For this review, use the dimensioned drawing (mm, ordinates from the lowest corner) and the shaded views. A direction names the side the tool comes from. Give positions to 0.01 mm unless a question says otherwise; leave off trailing zeros. Write each loop counter-clockwise with the first axis right and the second up, starting at its lowest first coordinate (ties: lowest second). Pieces come first, ordered by that corner, then holes. Notation, with made-up numbers: M 61.5,-3.5 L 90.5,-3.5 A15 ccw 90.5,6.5 Z; hole C 36.5,50 d9. An arc over 180 degrees is marked long. One line per item, written item: value. Start each with the question number.
Item 1: Consider section A-A, the plane x = 24. Write out the cut boundary in (y, z).
Item 2: Consider section D-D, the plane y = 47. Write out the cut boundary in (x, z).
Item 3: Clearance check with flat-ended pins moving along their axes: pin 1 Ø1.5 at (x, z) = (61, 39.5) entering from +Y; pin 2 Ø1 at (y, z) = (48.5, 64) entering from +X; pin 3 Ø8 at (x, y) = (54, 46) entering from +Z; pin 4 Ø8 at (x, z) = (66, 65) entering from -Y. State where each tip first meets the part, or that it passes through.
Item 4: Consider section B-B, the plane z = 16.5. Write out the cut boundary in (x, y).
Item 5: To check wall thickness, follow probe 1 along Z at (x, y) = (66, 22); probe 2 along Y at (x, z) = (16.5, 45.5); probe 3 along Y at (x, z) = (15, 66). State the ranges of each line that lie inside material, in increasing order.
Item 6: Consider section C-C, the plane y = 25. Write out the cut boundary in (x, z).
Item 7: Tool access review of the marked faces 1 and 2: name each direction out of +Z, -Z, +X, -X, +Y, -Y from which nothing blocks a thin tool from reaching the whole face with its end or side.
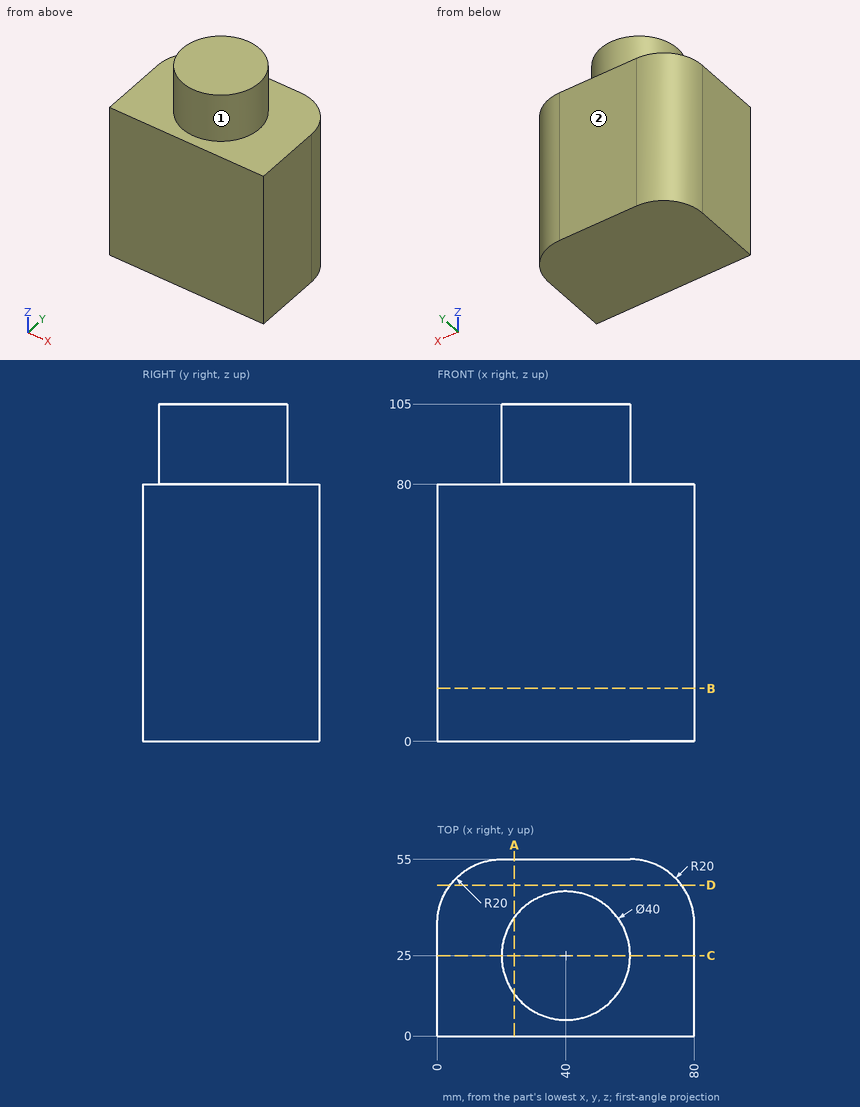
Model answer:
1. outline: M 0,0 L 55,0 L 55,80 L 37,80 L 37,105 L 13,105 L 13,80 L 0,80 Z
2. outline: M 4,0 L 76,0 L 76,80 L 4,80 Z
3. pin 1: stops at y = 55
3. pin 2: stops at x = 75.2
3. pin 3: stops at z = 80
3. pin 4: stops at y = 0
4. outline: M 0,0 L 80,0 L 80,35 A20 ccw 60,55 L 20,55 A20 ccw 0,35 Z
5. probe 1: z = 0 to 80
5. probe 2: y = 0 to 54.69
5. probe 3: y = 0 to 54.36
6. outline: M 0,0 L 80,0 L 80,80 L 60,80 L 60,105 L 20,105 L 20,80 L 0,80 Z
7. face 1: +Z
7. face 2: +Z, -Z, +X, -X, +Y
